from build123d import *

# Parameters (mm, degrees)
F1_DEPTH      = 2273.3
F3_DEPTH      = 508
F3_DEPTH_BACK = 50.8


with BuildPart() as f1:
    # F0 (on Right) → F1 (new body)
    with BuildSketch(Plane.YZ):
        with BuildLine():
            Line((-488.95, 736.6), (-488.95, 0))
            Line((-488.95, 0), (0, 0))
            Line((0, 0), (0, 113.825072))
            ThreePointArc((0, 113.825072), (23.140339, 186.915227), (84.128674, 233.370249))
            Line((84.128674, 233.370249), (363.629878, 333.605051))
            Line((363.629878, 333.605051), (361.486311, 339.58231))
            Line((361.486311, 339.58231), (0, 215.9))
            Line((0, 215.9), (0.10941, 365.604809))
            Line((0.10941, 365.604809), (0, 378.304337))
            Line((0, 378.304337), (0, 391.004337))
            Line((0, 391.004337), (0, 736.6))
            Line((0, 736.6), (-488.95, 736.6))
        make_face()
        Polygon((376.729838, 392.627121), (0, 391.004337), (0, 378.304337), (0.10941, 365.604809), (376.839247, 367.227592), (376.784543, 379.927357), align=None)
        Polygon((376.620426, 418.027003), (376.729838, 392.627121), (376.784543, 379.927357), (478.3836, 380.365), (478.3836, 389.89), align=None)
        Polygon((478.3836, 380.365), (376.784543, 379.927357), (376.839247, 367.227592), (376.948659, 341.82771), (478.465657, 370.840353), align=None)
    extrude(amount=F1_DEPTH)

    # F2 (on Front) → F3 (join, two sides)
    with BuildSketch(Plane.XZ) as f3_sk:
        Polygon((76.2, 0), (0, 0), (0, -50.8), (63.5, -50.8), (63.5, -25.4), (88.9, -25.4), (88.9, -50.8), (152.4, -50.8), (152.4, 0), align=None)
        Polygon((2273.3, -50.8), (2273.3, 0), (2197.1, 0), (2120.9, 0), (2120.9, -50.8), (2184.4, -50.8), (2184.4, -25.4), (2209.8, -25.4), (2209.8, -50.8), align=None)
    extrude(amount=F3_DEPTH)
    extrude(f3_sk.sketch, amount=-F3_DEPTH_BACK)


solid = f1.part
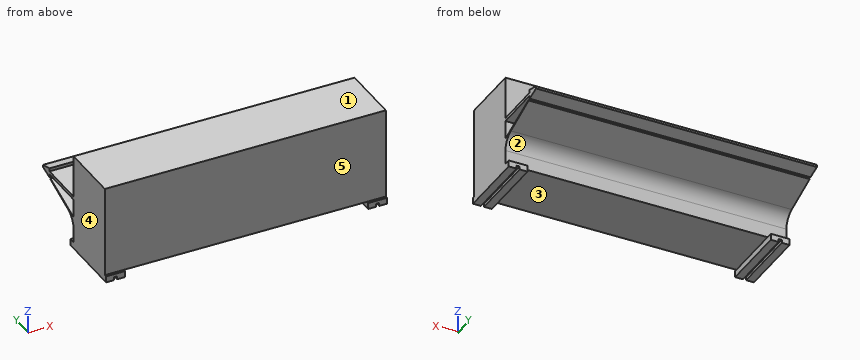
Geometry: final body of the model. Coordinates: model frame, mm. Face numbers are marked on the shaded views. A direction names the side the tool comes from. Round coordinates to 2 decimals unless told otherwise and drop trailing zeros. Loops run counter-clockwise (first coordinate to the right, second up) from the corner with the lowest first, then second, coordinate; pieces in that order, holes last. Notation, with made-up numbers: (0, 67.5) - (4, 67.5) arc R23 ccw to (4, 84.5) - close; hole circle Ø10 at (59, -25). An arc over 180 degrees is marked (long way). Write each question's results on one line, items separated by ' | '. Start each with the question number.
1) Access query for the marked faces 1 and 2. Directions: +Z, -Z, +X, -X, +Y, -Y. A direction counts if a zero-diameter tool reaches every point of the face in a straight line with its end or side. Return the directions, or none.
2) Cut plane B-B on y = -86.5. Return loops of the section in (x, z), then the cut area to 3 significant figures.
3) Cut plane C-C on y = 206. Return loops of the section in (x, z).
4) Line query: probe 1 along Y at (x, z) = (796, 434.5); probe 2 along Z at (x, y) = (1734, -361.5); probe 3 along X at (y, z) = (13, -9.5). Output: solid intervals per line, ascending. Write a range as [from, to].
5) First-contact query: P1, Ø15, axis at x = 2216.5, z = -36, coming from the +Y side; P2, Ø5.5, axis at x = 56, y = -494.5, coming from the +Z side; P3, Ø2, axis at x = 1588.5, z = 36.5, coming from the +Y side. Flat tips, straight axial feed; report the tip coordinate or a pass-through.
6) Cut plane A-A on x = 660.5. Return loops of the section in (y, z) (3 decimals), then the cut area to 3 significant figures.
7) Mould query, pull axis X, two halves, no side actions, for the marked faces 3, 4 and 5. Classes: released by +X, released by -X, zero draft, split by the parting line, or undercut.
8) Cut plane D-D on z = 676.5. Return loops of the section in (x, y).
Verdict:
1) face 1: +Z, +X, -X, +Y, -Y | face 2: +X, -X, +Y
2) outline: (0, -50.8) - (63.5, -50.8) - (63.5, -25.4) - (88.9, -25.4) - (88.9, -50.8) - (152.4, -50.8) - (152.4, 0) - (2120.9, 0) - (2120.9, -50.8) - (2184.4, -50.8) - (2184.4, -25.4) - (2209.8, -25.4) - (2209.8, -50.8) - (2273.3, -50.8) - (2273.3, 736.6) - (0, 736.6) - close | area: 1,690,000 mm2
3) outline: (0, 277.08) - (2273.3, 277.08) - (2273.3, 286.38) - (0, 286.38) - close; (0, 366.49) - (2273.3, 366.49) - (2273.3, 391.89) - (0, 391.89) - close
4) probe 1: y = [-488.95, 0] | probe 2: z = [0, 736.6] | probe 3: x = [0, 152.4], [2120.9, 2273.3]
5) P1: stops at y = 50.8 | P2: stops at z = 0 | P3: stops at y = 0
6) outline: (-488.95, 0) - (0, 0) - (0, 113.825) arc R127 cw to (84.129, 233.37) - (363.63, 333.605) - (361.486, 339.582) - (0, 215.9) - (0.109, 365.605) - (376.839, 367.228) - (376.949, 341.828) - (478.466, 370.84) - (478.384, 380.365) - (478.384, 389.89) - (376.62, 418.027) - (376.73, 392.627) - (0, 391.004) - (0, 736.6) - (-488.95, 736.6) - close | area: 380,000 mm2
7) face 3: undercut | face 4: released by -X | face 5: zero draft
8) outline: (0, -488.95) - (2273.3, -488.95) - (2273.3, 0) - (0, 0) - close
